Geometry: final body of the model. Coordinates: model frame, mm. Face numbers are marked on the shaded views. A direction names the side the tool comes from. Give positions to 0.01 mm unless a question says otherwise; leave off trailing zeros. Order: outer loops, then holes, each group sorted by start corner. A loop starts at its lowest first (then second) coordinate and runs counter-clockwise, first axis right, second up. Notation, with made-up numbers: (11.25, -39) -> (18.25, -39) arc R4 cw to (18.25, -34) -> close; hole circle Ø1 at (78.5, 33). An arc over 180 degrees is marked (long way). One line per question, with ' | ' between items. Start each with the question number.
(1) Ray query, L1, parallel to Z at x = 0, y = 36.4 (3 decimals); L2, parallel to Z at x = -31, y = 22.5; L3, parallel to X at y = 24.5, z = 1. Return the intervals inside material, ascending.
(2) Mould query, pull axis X, two halves, no side actions, for the marked faces 4, 5 and 6. Classes: +X half, -X half, draft (parallel to the pull), parting line (faces both ways), or undercut.
(3) Section A-A (x = -31). Return loops of the section in (y, z), then the cut area to 3 significant figures.
(4) Set-up query: the marked faces 1, 2 and 3. Return all of +Z, -Z, +X, -X, +Y, -Y with unobstructed straight access to the full face (end or side cutting, diameter ignored); none if empty.
(5) Section C-C (z = 1.5). State how many separate pieces and enclosed holes the cut face has, then the cut area to 3 significant figures.
(6) Section B-B (y = 24). Return loops of the section in (x, z).
(7) First-contact query: pin 1 Ø7.5 at (x, z) = (2.5, 1) entering from +Y; pin 2 Ø6 at (x, z) = (-29.5, 4.5) entering from -Y; pin 3 Ø6 at (y, z) = (15, -12) entering from +X; pin 4 Ø12 at (y, z) = (21.5, 2) entering from -X. Flat tips, straight axial feed; report the tip coordinate or a pass-through.
(8) Section D-D (y = 13). Return loops of the section in (x, z), then the cut area to 3 significant figures.
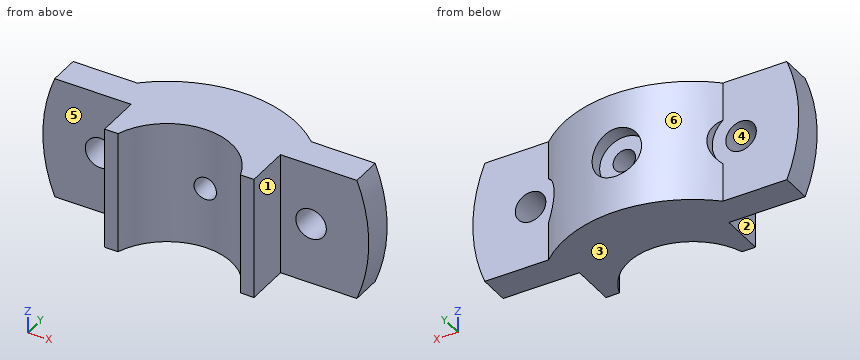
```python
from build123d import *

# Parameters (mm, degrees)
BOSS_EXTRUDE1_DEPTH                     = 18
CUT_EXTRUDE1_DEPTH                      = 9
SKETCH5_R                               = 4.5
CUT_EXTRUDE2_DEPTH                      = 10
CUT_EXTRUDE3_DEPTH                      = 10
CBORE_FOR_M6_HEX_HEAD_BOLT4_D           = 6.6
CBORE_FOR_M6_HEX_HEAD_BOLT4_CBORE_D     = 14.55
CBORE_FOR_M6_HEX_HEAD_BOLT4_CBORE_DEPTH = 4.38


with BuildPart() as part:
    # Sketch1 → Boss-Extrude1 (new body, symmetric)
    with BuildSketch(Plane.XY):
        with BuildLine():
            Line((18.027756377, 6), (22, 6))
            Line((22, 6), (22, 19))
            Line((22, 19), (50, 19))
            Line((50, 19), (50, 28))
            Line((50, 28), (29.380930315, 28))
            Line((29.380930315, 28), (25.690465157, 28))
            ThreePointArc((25.690465157, 28), (0, 38), (-25.690465157, 28))
            Line((-25.690465157, 28), (-29.380930315, 28))
            Line((-29.380930315, 28), (-50, 28))
            Line((-50, 28), (-50, 19))
            Line((-50, 19), (-22, 19))
            Line((-22, 19), (-22, 6))
            Line((-22, 6), (-18.027756377, 6))
            ThreePointArc((-18.027756377, 6), (0, 19), (18.027756377, 6))
        make_face()
    extrude(amount=BOSS_EXTRUDE1_DEPTH, both=True)

    # Sketch4 → Cut-Extrude1 (cut)
    with BuildSketch(Plane(origin=(0, 28, 0), x_dir=(1, 0, 0), z_dir=(0, 1, 0))):
        with BuildLine():
            Line((-44.497190923, 18), (-50, 18))
            Line((-50, 18), (-50, -18))
            Line((-50, -18), (-44.497190923, -18))
            ThreePointArc((-44.497190923, -18), (-48, 0), (-44.497190923, 18))
        make_face()
    cut_extrude1 = extrude(amount=-CUT_EXTRUDE1_DEPTH, mode=Mode.SUBTRACT)

    # Mirror1: Cut-Extrude1 across plane
    add(cut_extrude1.mirror(Plane(origin=(0, 0, 0), x_dir=(0, 0, 1), z_dir=(1, 0, 0))), mode=Mode.SUBTRACT)

    # Sketch5 → Cut-Extrude2 (cut)
    with BuildSketch(Plane(origin=(0, 28, 0), x_dir=(1, 0, 0), z_dir=(0, 1, 0))):
        with Locations(Location((-31, 0, 0), (0, 0, 180))):  # turned: the seam where the file's is
            Circle(SKETCH5_R)
    cut_extrude2 = extrude(amount=-CUT_EXTRUDE2_DEPTH, mode=Mode.SUBTRACT)

    # Sketch7 → Cut-Extrude3 (cut)
    with BuildSketch(Plane(origin=(0, 28, 0), x_dir=(1, 0, 0), z_dir=(0, 1, 0))):
        with BuildLine():
            Line((-25.690465157, -6.637683312), (-25.690465157, 6.637683312))
            ThreePointArc((-25.690465157, 6.637683312), (-22.5, 0), (-25.690465157, -6.637683312))
        make_face()
    cut_extrude3 = extrude(amount=CUT_EXTRUDE3_DEPTH, mode=Mode.SUBTRACT)

    # Mirror2: Cut-Extrude2, Cut-Extrude3 across plane
    add(cut_extrude2.mirror(Plane(origin=(0, 0, 0), x_dir=(0, 0, 1), z_dir=(1, 0, 0))), mode=Mode.SUBTRACT)
    add(cut_extrude3.mirror(Plane(origin=(0, 0, 0), x_dir=(0, 0, 1), z_dir=(1, 0, 0))), mode=Mode.SUBTRACT)

    # CBORE for M6 Hex Head Bolt4 (through all)
    with Locations(Plane(origin=(0, 38, 0), x_dir=(1, 0, 0), z_dir=(0, 1, 0))):
        with Locations((0, 0)):
            CounterBoreHole(CBORE_FOR_M6_HEX_HEAD_BOLT4_D / 2, CBORE_FOR_M6_HEX_HEAD_BOLT4_CBORE_D / 2, CBORE_FOR_M6_HEX_HEAD_BOLT4_CBORE_DEPTH)


solid = part.part
```
Response:
1) L1: z = -18 to -7.275, 7.275 to 18 | L2: z = -18 to -4.5, 4.5 to 18 | L3: x = -47.99 to -35.39, -26.61 to -3.14, 3.14 to 26.61, 35.39 to 47.99
2) face 4: undercut | face 5: draft | face 6: parting line
3) outline: (19, -18) -> (28, -18) -> (28, -4.5) -> (19, -4.5) -> close; (19, 4.5) -> (28, 4.5) -> (28, 18) -> (19, 18) -> close | area: 243 mm^2
4) face 1: +Z, -Z, +X, -Y | face 2: +Z, -Z, -X, -Y | face 3: -Z, +X, -X, +Y, -Y
5) separate pieces: 4 | enclosed holes: 0 | area: 1,140 mm^2
6) outline: (-44.5, -18) -> (44.5, -18) arc R48 ccw to (44.5, 18) -> (-44.5, 18) arc R48 ccw to start; hole circle Ø9 at (-31, 0); hole circle Ø6.6 at (0, 0); hole circle Ø9 at (31, 0)
7) pin 1: stops at y = 33.62 | pin 2: stops at y = 19 | pin 3: stops at x = 22 | pin 4: stops at x = -48
8) outline: (-22, -18) -> (-13.86, -18) -> (-13.86, 18) -> (-22, 18) -> close; (13.86, -18) -> (22, -18) -> (22, 18) -> (13.86, 18) -> close | area: 586 mm^2
